from build123d import *

# Parameters (mm, degrees)
F1_DEPTH = 6.35


with BuildPart() as f1:
    # F0 (on Top) → F1 (new body)
    with BuildSketch(Plane.XY):
        with BuildLine():
            Line((-14.298079, -8.255), (0, 0))
            Line((0, 0), (0, 16.51))
            ThreePointArc((0, 16.51), (-6.985, 18.381625), (-12.098375, 23.495))
            ThreePointArc((-12.098375, 23.495), (-9.886492, 15.204646), (-12.13386, 6.923841))
            ThreePointArc((-12.13386, 6.923841), (-18.172091, 0.924276), (-26.396454, -1.27))
            ThreePointArc((-26.396454, -1.27), (-25.702754, -1.287234), (-25.010766, -1.338893))
            ThreePointArc((-25.010766, -1.338893), (-18.819309, -3.5034), (-14.298079, -8.255))
        make_face()
        with BuildLine():
            Line((0, -13.97), (0, 0))
            Line((0, 0), (-14.298079, -8.255))
            ThreePointArc((-14.298079, -8.255), (-12.902471, -11.624298), (-12.426454, -15.24))
            ThreePointArc((-12.426454, -15.24), (-12.902471, -18.855702), (-14.298079, -22.225))
            ThreePointArc((-14.298079, -22.225), (-8.255, -16.181921), (0, -13.97))
        make_face()
        with BuildLine():
            Line((12.098375, 6.985), (0, 0))
            Line((0, 0), (14.298079, -8.255))
            ThreePointArc((14.298079, -8.255), (19.411454, -3.141625), (26.396454, -1.27))
            ThreePointArc((26.396454, -1.27), (18.141454, 0.941921), (12.098375, 6.985))
        make_face()
        with BuildLine():
            Line((14.298079, -8.255), (0, 0))
            Line((0, 0), (0, -13.97))
            ThreePointArc((0, -13.97), (8.255, -16.181921), (14.298079, -22.225))
            ThreePointArc((14.298079, -22.225), (12.426454, -15.24), (14.298079, -8.255))
        make_face()
        with BuildLine():
            Line((0, 16.51), (0, 0))
            Line((0, 0), (12.098375, 6.985))
            ThreePointArc((12.098375, 6.985), (9.886454, 15.24), (12.098375, 23.495))
            ThreePointArc((12.098375, 23.495), (6.985, 18.381625), (0, 16.51))
        make_face()
        with BuildLine():
            ThreePointArc((11.049, 30.48), (-7.812823, 38.292823), (0, 19.431))
            ThreePointArc((0, 19.431), (7.812823, 22.667177), (11.049, 30.48))
        make_face()
        with BuildLine():
            ThreePointArc((-12.098375, 23.495), (-6.985, 18.381625), (0, 16.51))
            ThreePointArc((0, 16.51), (6.985, 18.381625), (12.098375, 23.495))
            ThreePointArc((12.098375, 23.495), (13.493984, 26.864298), (13.97, 30.48))
            ThreePointArc((13.97, 30.48), (10.291919, 39.92655), (1.194438, 44.398844))
            ThreePointArc((1.194438, 44.398844), (-1.30857, 44.263376), (-3.792353, 43.925407))
            ThreePointArc((-3.792353, 43.925407), (-12.941375, 35.741341), (-12.098375, 23.495))
        make_face()
        with BuildLine():
            ThreePointArc((11.049, 30.48), (7.812823, 22.667177), (0, 19.431))
            ThreePointArc((0, 19.431), (-7.812823, 38.292823), (11.049, 30.48))
        make_face(mode=Mode.SUBTRACT)
        with BuildLine():
            ThreePointArc((-15.347454, -15.24), (-15.72394, -12.380308), (-16.82774, -9.7155))
            ThreePointArc((-16.82774, -9.7155), (-37.068969, -18.099692), (-15.347454, -15.24))
        make_face()
        with BuildLine():
            ThreePointArc((-12.426454, -15.24), (-12.902471, -11.624298), (-14.298079, -8.255))
            ThreePointArc((-14.298079, -8.255), (-18.819309, -3.5034), (-25.010766, -1.338893))
            ThreePointArc((-25.010766, -1.338893), (-26.431469, -1.403743), (-27.852483, -1.346085))
            ThreePointArc((-27.852483, -1.346085), (-38.559988, -8.369094), (-39.047746, -21.165008))
            ThreePointArc((-39.047746, -21.165008), (-37.678923, -23.264942), (-36.144342, -25.246977))
            ThreePointArc((-36.144342, -25.246977), (-24.482222, -29.07823), (-14.298079, -22.225))
            ThreePointArc((-14.298079, -22.225), (-12.902471, -18.855702), (-12.426454, -15.24))
        make_face()
        with BuildLine():
            ThreePointArc((-15.347454, -15.24), (-37.068969, -18.099692), (-16.82774, -9.7155))
            ThreePointArc((-16.82774, -9.7155), (-15.72394, -12.380308), (-15.347454, -15.24))
        make_face(mode=Mode.SUBTRACT)
        with BuildLine():
            ThreePointArc((37.445454, -15.24), (29.256146, -4.567486), (16.82774, -9.7155))
            ThreePointArc((16.82774, -9.7155), (23.536763, -25.912514), (37.445454, -15.24))
        make_face()
        with BuildLine():
            ThreePointArc((26.396454, -1.27), (19.411454, -3.141625), (14.298079, -8.255))
            ThreePointArc((14.298079, -8.255), (12.426454, -15.24), (14.298079, -22.225))
            ThreePointArc((14.298079, -22.225), (25.798688, -29.197205), (37.853308, -23.233836))
            ThreePointArc((37.853308, -23.233836), (38.987493, -20.998433), (39.936694, -18.678429))
            ThreePointArc((39.936694, -18.678429), (40.258598, -16.972591), (40.366454, -15.24))
            ThreePointArc((40.366454, -15.24), (36.274736, -5.361718), (26.396454, -1.27))
        make_face()
        with BuildLine():
            ThreePointArc((37.445454, -15.24), (23.536763, -25.912514), (16.82774, -9.7155))
            ThreePointArc((16.82774, -9.7155), (29.256146, -4.567486), (37.445454, -15.24))
        make_face(mode=Mode.SUBTRACT)
        with BuildLine():
            ThreePointArc((-23.504818, 31.494801), (-16.916434, 28.757001), (-12.098375, 23.495))
            ThreePointArc((-12.098375, 23.495), (-12.941375, 35.741341), (-3.792353, 43.925407))
            ThreePointArc((-3.792353, 43.925407), (-14.865803, 39.640368), (-23.504818, 31.494801))
        make_face()
        with BuildLine():
            ThreePointArc((-27.852483, -1.346085), (-26.431469, -1.403743), (-25.010766, -1.338893))
            ThreePointArc((-25.010766, -1.338893), (-25.702754, -1.287234), (-26.396454, -1.27))
            ThreePointArc((-26.396454, -1.27), (-27.125462, -1.289034), (-27.852483, -1.346085))
        make_face()
        with BuildLine():
            ThreePointArc((39.027706, 4.608369), (33.362511, 0.271561), (26.396454, -1.27))
            ThreePointArc((26.396454, -1.27), (36.274736, -5.361718), (40.366454, -15.24))
            ThreePointArc((40.366454, -15.24), (40.258598, -16.972591), (39.936694, -18.678429))
            ThreePointArc((39.936694, -18.678429), (41.762467, -6.946021), (39.027706, 4.608369))
        make_face()
        with BuildLine():
            ThreePointArc((-15.522888, -36.10317), (-16.446076, -29.028562), (-14.298079, -22.225))
            ThreePointArc((-14.298079, -22.225), (-24.482222, -29.07823), (-36.144342, -25.246977))
            ThreePointArc((-36.144342, -25.246977), (-26.896664, -32.694347), (-15.522888, -36.10317))
        make_face()
        with BuildLine():
            ThreePointArc((-1.194438, 44.398844), (-2.504607, 44.223647), (-3.792353, 43.925407))
            ThreePointArc((-3.792353, 43.925407), (-1.30857, 44.263376), (1.194438, 44.398844))
            ThreePointArc((1.194438, 44.398844), (0, 44.414908), (-1.194438, 44.398844))
        make_face()
        with BuildLine():
            ThreePointArc((39.936694, -18.678429), (38.987493, -20.998433), (37.853308, -23.233836))
            ThreePointArc((37.853308, -23.233836), (39.100847, -21.050275), (39.936694, -18.678429))
        make_face()
        with BuildLine():
            ThreePointArc((-37.853308, -23.233836), (-37.046498, -24.280877), (-36.144342, -25.246977))
            ThreePointArc((-36.144342, -25.246977), (-37.678923, -23.264942), (-39.047746, -21.165008))
            ThreePointArc((-39.047746, -21.165008), (-38.464438, -22.207454), (-37.853308, -23.233836))
        make_face()
        with BuildLine():
            ThreePointArc((1.194438, 44.398844), (0, 44.45), (-1.194438, 44.398844))
            ThreePointArc((-1.194438, 44.398844), (0, 44.414908), (1.194438, 44.398844))
        make_face()
        with BuildLine():
            ThreePointArc((-37.853308, -23.233836), (-38.464438, -22.207454), (-39.047746, -21.165008))
            ThreePointArc((-39.047746, -21.165008), (-38.494829, -22.225), (-37.853308, -23.233836))
        make_face()
    extrude(amount=F1_DEPTH)


solid = f1.part
Verification items for the finished model (mm, model axes). Give positions to 0.01 mm unless a question says otherwise; leave off trailing zeros. Write each loop counter-clockwise with the first axis right and the second up, starting at its lowest first coordinate (ties: lowest second). Pieces come first, ordered by that corner, then holes. Notation, with made-up numbers: (4.5, 8) - (26.5, 8) arc R26 cw to (26.5, 23) - close; hole circle Ø9 at (89.25, 27). An arc over 180 degrees is marked (long way). Answer as CSV lines item,"result". Start each with the question number.
1. Sectioned sample at C-C (x = 2.5). Record the boundary of the cut face in (y, z), then the cut area to 3 significant figures.
2. Sectioned sample at A-A (z = 1.25). Record the boundary of the cut face in (x, y) (1 decimal).
3. Thickness scan on line 1 (Y direction, x = -21, z = 2.5); line 2 (X direction, y = -8, z = 4); line 3 (Y direction, x = -8, z = 2.25). Record the ranges inside material, lowest first.
4. Sectioned sample at B-B (y = -28). Record the boundary of the cut face in (x, z), then the cut area to 3 significant figures.
5. Sectioned sample at D-D (y = 8.5). Record the boundary of the cut face in (x, z), then the cut area to 3 significant figures.
6. Depth check by flat-ended pin: pin 1 (1.5 mm diameter, centred on x = 31.5, z = 2, fed in from +Y); pin 2 (3 mm diameter, centred on x = -12, z = 4.5, fed in from -Y); pin 3 (20 mm diameter, centred on x = -26.4, y = -15.24, fed in from +Z). Enter the tip coordinate at first touch or a pass-through.
Derived:
1,outline,"(-14.16, 0) - (19.72, 0) - (19.72, 6.35) - (-14.16, 6.35) - close; (41.24, 0) - (44.22, 0) - (44.22, 6.35) - (41.24, 6.35) - close"
1,area,"234 mm²"
2,outline,"(-39, -21.2) arc R14 ccw to (-37.9, -23.2) arc R14 ccw to (-36.1, -25.2) arc R30.9 ccw to (-15.5, -36.1) arc R16.5 cw to (0, -14) arc R16.5 cw to (14.3, -22.2) arc R14 ccw to (37.9, -23.2) arc R14 ccw to (39.9, -18.7) arc R30.9 ccw to (39, 4.6) arc R16.5 cw to (26.4, -1.3) arc R16.5 cw to (12.1, 7) arc R16.5 cw to (12.1, 23.5) arc R14 ccw to (14, 30.5) arc R14 ccw to (1.2, 44.4) arc R14 ccw to (-1.2, 44.4) arc R14 ccw to (-3.8, 43.9) arc R30.9 ccw to (-23.5, 31.5) arc R16.5 cw to (-12.1, 23.5) arc R16.5 cw to (-12.1, 6.9) arc R16.5 cw to (-26.4, -1.3) arc R14 ccw to (-27.9, -1.3) arc R14 ccw to start; hole circle Ø22.1 at (-26.4, -15.2); hole circle Ø22.1 at (0, 30.5); hole circle Ø22.1 at (26.4, -15.2)"
3,line 1,"-35.06 to -24.88, -5.6 to -0.36, 30.84 to 34.56"
3,line 2,"-38.34 to -34.74, -18.05 to 18.05, 34.74 to 41.79"
3,line 3,"-16.04 to 22.86, 38.1 to 42.87"
4,outline,"(-33.52, 0) - (-16.32, 0) - (-16.32, 6.35) - (-33.52, 6.35) - close; (20.71, 0) - (32.08, 0) - (32.08, 6.35) - (20.71, 6.35) - close"
4,area,"181 mm²"
5,outline,"(-11.32, 0) - (11.32, 0) - (11.32, 6.35) - (-11.32, 6.35) - close"
5,area,"144 mm²"
6,pin 1,"y = -0.2"
6,pin 2,"y = -20.98"
6,pin 3,"through"
